Part model, mm, in its own coordinate system. Round coordinates to 2 decimals unless told otherwise and drop trailing zeros. Loops run counter-clockwise (first coordinate to the right, second up) from the corner with the lowest first, then second, coordinate; pieces in that order, holes last.
1) Probe line 1 (Y direction, x = 35.85, z = 11.25); line 2 (X direction, y = 18.5, z = 10); line 3 (Y direction, x = 20.35, z = 11.25). List the from-to ranges inside material, lowest first.
2) Drop a flat-ended pin along its axis: P1, Ø1, axis at x = 19, y = 25, coming from the +Z side. Give the stop position or say it passes through.
3) Band-saw the part on D-D, the plane y = 25.25. Write the cut outline in (x, z).
4) Band-saw the part on A-A, the plane y = 5.35. Write the cut outline in (x, z).
5) Band-saw the part on C-C, the plane x = 35.85. Write the cut outline in (y, z).
6) Mould opens along X. For faces 1 (the flat face through (40.7, 14, 8)), 2 (the flat face through (0, 14, 8)), 3 (the flat face through (20, 11, 15.8)), 4 (the cylindrical face through (3.25, 5.42, 8.01)) say: +X half, -X half, draft (parallel to the pull), parting line (faces both ways), or undercut.
7) Band-saw the part on B-B, the plane z = 1. Write the cut outline in (x, y).
from build123d import *

# Parameters (mm, degrees)
SKETCH_1_W          = 40.7
SKETCH_1_H          = 28.6
EXTRUDE_1_DEPTH     = 15.8
SKETCH_2_R          = 1.6
SKETCH_2_R_2        = 6.3
CUT_EXTRUDE_1_DEPTH = 53.192815598
SKETCH_3_R          = 1
CUT_EXTRUDE_2_DEPTH = 53.192815598


with BuildPart() as part:
    # Эскиз1 → Бобышка-Вытянуть1 (new body)
    with BuildSketch(Plane.XY):
        with Locations((20.35, 14.3)):
            Rectangle(SKETCH_1_W, SKETCH_1_H)
    extrude(amount=EXTRUDE_1_DEPTH)

    # Эскиз2 → Вырез-Вытянуть1 (cut, through all)
    with BuildSketch(Plane.XY.offset(15.8)):
        with Locations((35.85, 5.35)):
            Circle(SKETCH_2_R)
        with Locations((4.85, 5.35)):
            Circle(SKETCH_2_R)
        with Locations((20.35, 20.3)):
            Circle(SKETCH_2_R_2)
    extrude(amount=-CUT_EXTRUDE_1_DEPTH, mode=Mode.SUBTRACT)

    # Эскиз3 → Вырез-Вытянуть2 (cut, through all)
    with BuildSketch(Plane.XZ):
        with Locations(Location((14.2, 10, 0), (0, 0, 270))):
            Circle(SKETCH_3_R)
        with Locations(Location((26.5, 10, 0), (0, 0, 270))):
            Circle(SKETCH_3_R)
    extrude(amount=-CUT_EXTRUDE_2_DEPTH, mode=Mode.SUBTRACT)


solid = part.part
Reported:
1. line 1: y = 0 to 3.75, 6.95 to 28.6
1. line 2: x = 0 to 13.2, 27.5 to 40.7
1. line 3: y = 0 to 14, 26.6 to 28.6
2. P1: passes through
3. outline: (0, 0) - (16.45, 0) - (16.45, 15.8) - (0, 15.8) - close; (24.25, 0) - (40.7, 0) - (40.7, 15.8) - (24.25, 15.8) - close; hole circle Ø2 at (14.2, 10); hole circle Ø2 at (26.5, 10)
4. outline: (0, 0) - (3.25, 0) - (3.25, 15.8) - (0, 15.8) - close; (6.45, 0) - (34.25, 0) - (34.25, 15.8) - (6.45, 15.8) - close; (37.45, 0) - (40.7, 0) - (40.7, 15.8) - (37.45, 15.8) - close; hole circle Ø2 at (14.2, 10); hole circle Ø2 at (26.5, 10)
5. outline: (0, 0) - (3.75, 0) - (3.75, 15.8) - (0, 15.8) - close; (6.95, 0) - (28.6, 0) - (28.6, 15.8) - (6.95, 15.8) - close
6. face 1: +X half
6. face 2: -X half
6. face 3: draft
6. face 4: undercut
7. outline: (0, 0) - (40.7, 0) - (40.7, 28.6) - (0, 28.6) - close; hole circle Ø3.2 at (4.85, 5.35); hole circle Ø12.6 at (20.35, 20.3); hole circle Ø3.2 at (35.85, 5.35)
